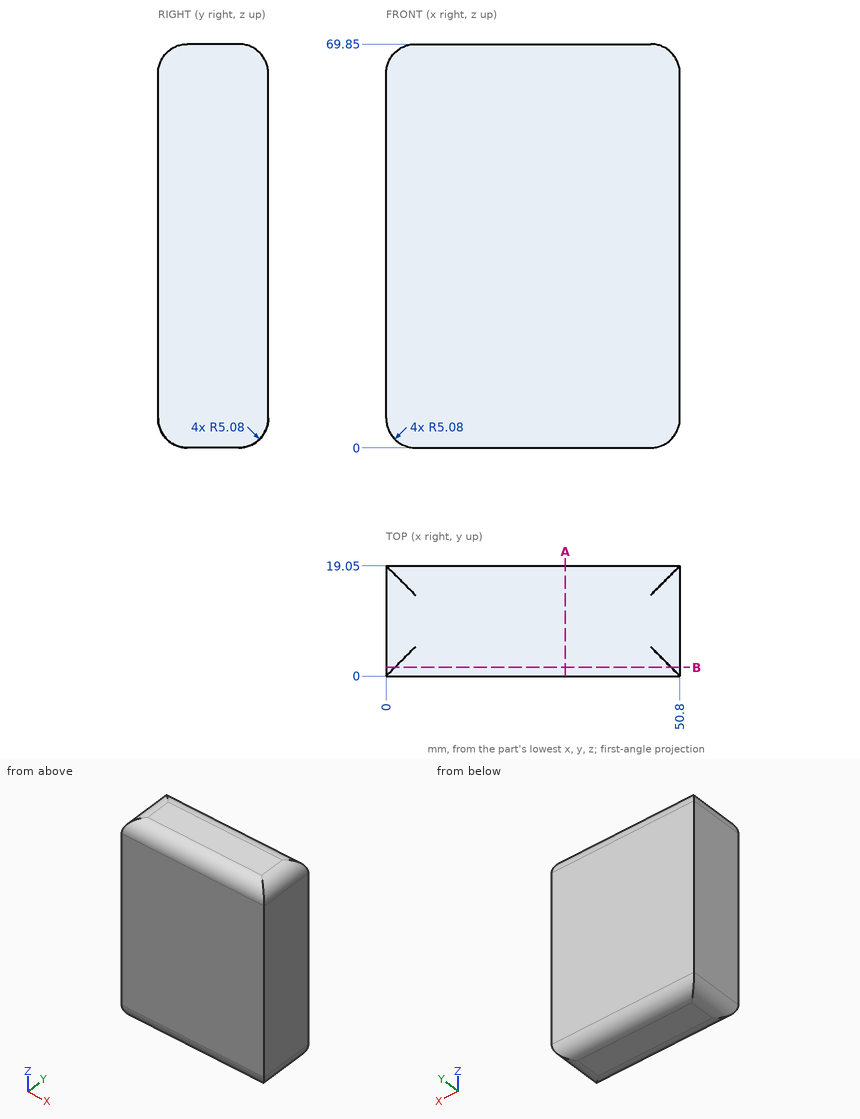
Drawing for the job (mm, zero at the part's lowest x, y, z). Give positions to 0.01 mm unless a question says otherwise; leave off trailing zeros. Loops run counter-clockwise (first coordinate to the right, second up) from the corner with the lowest first, then second, coordinate; pieces in that order, holes last. Notation, with made-up numbers: (-13, 40) - (43, 40) arc R13 cw to (43, 64) - close; hole circle Ø7 at (17, -31.75). An arc over 180 degrees is marked (long way). Write item = value, one per line. Start each with the question number.
1) Probe probe 1 along Z at (x, y) = (24, 2.5); probe 2 along X at (y, z) = (10, 3.5); probe 3 along Y at (x, z) = (27.5, 65.5). List the from-to ranges inside material, lowest first. Write a range as from..to.
2) Band-saw the part on A-A on x = 31. Give the cut face in (y, z), plus the area to 3 significant figures.
3) Band-saw the part on B-B on y = 1.5. Give the cut face in (x, z).
Final values:
q1.probe_1 = 0.7..69.15
q1.probe_2 = 0.25..50.55
q1.probe_3 = 0.05..19
q2.outline = (0, 5.08) arc R5.08 ccw to (5.08, 0) - (13.97, 0) arc R5.08 ccw to (19.05, 5.08) - (19.05, 64.77) arc R5.08 ccw to (13.97, 69.85) - (5.08, 69.85) arc R5.08 ccw to (0, 64.77) - close
q2.area = 1,310 mm²
q3.outline = (0, 5.08) arc R5.08 ccw to (1.5, 1.48) - (49.3, 1.48) arc R5.08 ccw to (50.8, 5.08) - (50.8, 64.77) arc R5.08 ccw to (49.3, 68.37) - (1.5, 68.37) arc R5.08 ccw to (0, 64.77) - close
